For this review, take the finished solid that the model builds, in its own axes (mm). Face numbers are marked on the shaded views. A direction names the side the tool comes from. Coordinates: 2 decimals unless noted, no trailing zeros. Loops run counter-clockwise (first coordinate to the right, second up) from the corner with the lowest first, then second, coordinate; pieces in that order, holes last. Notation, with made-up numbers: M 54.5,36 L 98.5,36 A33 ccw 98.5,73 Z; hole C -31.5,7 d10. An arc over 180 degrees is marked long. Write each question's results on one line, items separated by ' | '. Start each with the question number.
```python
from build123d import *

# Parameters (mm, degrees)
SKETCH1_W                      = 41.4
SKETCH1_H                      = 33.02
SKETCH1_R                      = 3.175
BOSS_EXTRUDE1_DEPTH            = 12
SKETCH2_W                      = 41.4
SKETCH2_H                      = 7.62
BOSS_EXTRUDE2_DEPTH            = 53
CUT_EXTRUDE1_REACH             = 72.186
SKETCH4_R                      = 3.175
CUT_EXTRUDE1_DIRECTION_2_REACH = 72.186
CUT_EXTRUDE3_REACH             = 72.186
CUT_EXTRUDE3_DIRECTION_2_REACH = 72.186
FILLET1_R                      = 10


with BuildPart() as part:
    # Sketch1 → Boss-Extrude1 (new body)
    with BuildSketch(Plane.XY):
        Rectangle(SKETCH1_W, SKETCH1_H)
        with Locations((12.7, 0)):
            Circle(SKETCH1_R, mode=Mode.SUBTRACT)
        with Locations((-12.7, 0)):
            Circle(SKETCH1_R, mode=Mode.SUBTRACT)
    extrude(amount=BOSS_EXTRUDE1_DEPTH)

    # Sketch2 → Boss-Extrude2 (add)
    with BuildSketch(Plane.XY.offset(12)):
        with Locations((0, 12.7)):
            Rectangle(SKETCH2_W, SKETCH2_H)
        with Locations((0, -12.7)):
            Rectangle(SKETCH2_W, SKETCH2_H)
    extrude(amount=BOSS_EXTRUDE2_DEPTH)

    # Cut-Extrude1: up to this face of the body (flat: up to its plane)
    cut_extrude1_end = Plane(part.part.faces().sort_by_distance((0, -16.51, 32.5))[0])
    # Sketch4 → Cut-Extrude1 (cut, up to the picked face)
    with BuildSketch(Plane(origin=(0, 0, 0), x_dir=(1, 0, 0), z_dir=(0, 1, 0)), mode=Mode.PRIVATE) as cut_extrude1_sk1:
        with Locations(Location((0, -35.5, 0), (0, 0, 270))):
            Circle(SKETCH4_R)
    cut_extrude1_tool1 = split(extrude(cut_extrude1_sk1.sketch, amount=-CUT_EXTRUDE1_REACH, mode=Mode.PRIVATE), bisect_by=cut_extrude1_end, keep=Keep.BOTH, mode=Mode.PRIVATE)
    add(cut_extrude1_tool1.solids().sort_by(Axis((0, 0, 35.5), (0, -1, 0)))[0], mode=Mode.SUBTRACT)

    # Cut-Extrude1 direction 2: up to this face of the body (flat: up to its plane)
    cut_extrude1_direction_2_end = Plane(part.part.faces().sort_by_distance((0, 16.51, 32.5))[0])
    # Sketch4 → Cut-Extrude1 direction 2 (cut, up to the picked face)
    with BuildSketch(Plane(origin=(0, 0, 0), x_dir=(1, 0, 0), z_dir=(0, 1, 0)), mode=Mode.PRIVATE) as cut_extrude1_direction_2_sk1:
        with Locations(Location((0, -35.5, 0), (0, 0, 270))):
            Circle(SKETCH4_R)
    cut_extrude1_direction_2_tool1 = split(extrude(cut_extrude1_direction_2_sk1.sketch, amount=CUT_EXTRUDE1_DIRECTION_2_REACH, mode=Mode.PRIVATE), bisect_by=cut_extrude1_direction_2_end, keep=Keep.BOTH, mode=Mode.PRIVATE)
    add(cut_extrude1_direction_2_tool1.solids().sort_by(Axis((0, 0, 35.5), (0, 1, 0)))[0], mode=Mode.SUBTRACT)

    # Cut-Extrude3: up to this face of the body (flat: up to its plane)
    cut_extrude3_end = Plane(part.part.faces().sort_by_distance((-19.929353518, -16.51, 32.5))[0])
    # Sketch6 → Cut-Extrude3 (cut, up to the picked face)
    with BuildSketch(Plane(origin=(0, 0, 0), x_dir=(1, 0, 0), z_dir=(0, 1, 0)), mode=Mode.PRIVATE) as cut_extrude3_sk1:
        with BuildLine():
            Line((-8, -35.5), (-8, -20))
            ThreePointArc((-8, -20), (-10.343145751, -14.343145751), (-16, -12))
            Line((-16, -12), (-20.7, -12))
            Line((-20.7, -12), (-20.7, -65))
            Line((-20.7, -65), (20.7, -65))
            Line((20.7, -65), (20.7, -12))
            Line((20.7, -12), (16, -12))
            ThreePointArc((16, -12), (10.343145751, -14.343145751), (8, -20))
            Line((8, -20), (8, -35.5))
            ThreePointArc((8, -35.5), (0, -43.5), (-8, -35.5))
        make_face()
    cut_extrude3_tool1 = split(extrude(cut_extrude3_sk1.sketch, amount=-CUT_EXTRUDE3_REACH, mode=Mode.PRIVATE), bisect_by=cut_extrude3_end, keep=Keep.BOTH, mode=Mode.PRIVATE)
    add(cut_extrude3_tool1.solids().sort_by(Axis((-8.67253, 0, 27.75), (0, -1, 0)))[0], mode=Mode.SUBTRACT)

    # Cut-Extrude3 direction 2: up to this face of the body (flat: up to its plane)
    cut_extrude3_direction_2_end = Plane(part.part.faces().sort_by_distance((19.929353518, 16.51, 32.5))[0])
    # Sketch6 → Cut-Extrude3 direction 2 (cut, up to the picked face)
    with BuildSketch(Plane(origin=(0, 0, 0), x_dir=(1, 0, 0), z_dir=(0, 1, 0)), mode=Mode.PRIVATE) as cut_extrude3_direction_2_sk1:
        with BuildLine():
            Line((-8, -35.5), (-8, -20))
            ThreePointArc((-8, -20), (-10.343145751, -14.343145751), (-16, -12))
            Line((-16, -12), (-20.7, -12))
            Line((-20.7, -12), (-20.7, -65))
            Line((-20.7, -65), (20.7, -65))
            Line((20.7, -65), (20.7, -12))
            Line((20.7, -12), (16, -12))
            ThreePointArc((16, -12), (10.343145751, -14.343145751), (8, -20))
            Line((8, -20), (8, -35.5))
            ThreePointArc((8, -35.5), (0, -43.5), (-8, -35.5))
        make_face()
    cut_extrude3_direction_2_tool1 = split(extrude(cut_extrude3_direction_2_sk1.sketch, amount=CUT_EXTRUDE3_DIRECTION_2_REACH, mode=Mode.PRIVATE), bisect_by=cut_extrude3_direction_2_end, keep=Keep.BOTH, mode=Mode.PRIVATE)
    add(cut_extrude3_direction_2_tool1.solids().sort_by(Axis((-8.67253, 0, 27.75), (0, 1, 0)))[0], mode=Mode.SUBTRACT)

    # Fillet1
    fillet1_edges = [part.edges().sort_by_distance(p)[0] for p in [
        (-20.7, -16.51, 6),
        (-20.7, 16.51, 6),
        (20.7, -16.51, 6),
        (20.7, 16.51, 6),
    ]]
    fillet(fillet1_edges, radius=FILLET1_R)


solid = part.part
```
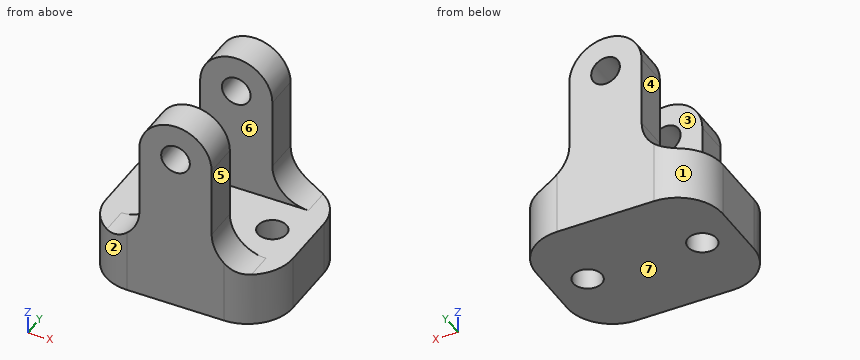
Q1. Take a section at D-D, the plane z = 26.5. Give the boundary of the cut face in (x, y).
Q2. The part is to be moulded in two halves that separate along Y. For the marked faces 1, 2, 3 and 4, say which applies: pulls with the +Y half, pulls with the -Y half, needs draft (parallel to the pull), parting line crosses it, or undercut.
Q3. Take a section at B-B, the plane x = 0. Give the boundary of the cut face in (y, z) (3 decimals).
Q4. To check wall thickness, follow line 1 along Y through (x, z) = (-4.5, 18.5); line 2 along X through (y, z) = (11, 35.5) (3 decimals); line 3 along Z through (x, y) = (10.5, 2.5). State the ranges of each line that lie inside material, in increasing order.
Q5. Take a section at A-A, the plane y = 0. Give the boundary of the cut face in (x, z) (3 decimals).
Q6. For the marked faces 5, 6 and 7, list the 3-axis set-ups (+Z, -Z, +X, -X, +Y, -Y) from which the entire face can be reached by the end or side of a thin tool; tool diameter is ignored.
Q7. Take a section at C-C, the plane z = 10. Give the boundary of the cut face in (x, y) (3 decimals).
Q8. Insertion check: P1, Ø4, axis at y = -9.5, z = 8, coming from the +X side; P2, Ø2.5, axis at y = 14.5, z = 25, coming from the -X side; P3, Ø2.5, axis at y = -14, z = 26.5, coming from the +X side. Each pin has a flat end and moves straight along its axis. Give the tip position at first contact, or say it passes through.
Results:
1) outline: M -8,-16.51 L 8,-16.51 L 8,-8.89 L -8,-8.89 Z; M -8,8.89 L 8,8.89 L 8,16.51 L -8,16.51 Z
2) face 1: pulls with the +Y half | face 2: pulls with the -Y half | face 3: undercut | face 4: needs draft
3) outline: M -16.51,0 L 16.51,0 L 16.51,32.325 L 8.89,32.325 L 8.89,12 L -8.89,12 L -8.89,32.325 L -16.51,32.325 Z; M -16.51,38.675 L -8.89,38.675 L -8.89,43.5 L -16.51,43.5 Z; M 8.89,38.675 L 16.51,38.675 L 16.51,43.5 L 8.89,43.5 Z
4) line 1: -16.51 to -8.89, 8.89 to 16.51 | line 2: -8 to -3.175, 3.175 to 8 | line 3: 0 to 12
5) outline: M -20.7,0 L -15.875,0 L -15.875,12 L -20.7,12 Z; M -9.525,0 L 9.525,0 L 9.525,12 L -9.525,12 Z; M 15.875,0 L 20.7,0 L 20.7,12 L 15.875,12 Z
6) face 5: +Z, +X, +Y, -Y | face 6: +Z, +X, -X | face 7: -Z, +X, -X, +Y, -Y
7) outline: M -20.7,-6.51 A10 ccw -10.7,-16.51 L 10.7,-16.51 A10 ccw 20.7,-6.51 L 20.7,6.51 A10 ccw 10.7,16.51 L -10.7,16.51 A10 ccw -20.7,6.51 Z; hole C -12.7,0 d6.35; hole C 12.7,0 d6.35
8) P1: x = 20.65 | P2: x = -8 | P3: x = 8
